```python
from build123d import *

# Parameters (mm, degrees)
SKETCH_1_W          = 120
SKETCH_1_H          = 64.5
EXTRUDE_1_DEPTH     = 44.5
SKETCH_2_W          = 24.5
SKETCH_2_H          = 24.5
CUT_EXTRUDE_1_DEPTH = 121
EXTRUDE_2_DEPTH     = 64.5
SKETCH_4_R          = 20
EXTRUDE_3_DEPTH     = 30
SKETCH_5_R          = 20
EXTRUDE_4_DEPTH     = 30
SKETCH_6_W          = 64.5
SKETCH_6_H          = 20
EXTRUDE_5_DEPTH     = 120


with BuildPart() as part:
    # 草图1 → 凸台-拉伸1 (new body)
    with BuildSketch(Plane(origin=(0, 0, 0), x_dir=(1, 0, 0), z_dir=(0, 1, 0))):
        Rectangle(SKETCH_1_W, SKETCH_1_H)
    extrude(amount=EXTRUDE_1_DEPTH)

    # 草图2 → 切除-拉伸1 (cut, through all)
    with BuildSketch(Plane(origin=(60, 0, 0), x_dir=(0, 0, -1), z_dir=(1, 0, 0))):
        with Locations((0, 12.25)):
            Rectangle(SKETCH_2_W, SKETCH_2_H)
    extrude(amount=-CUT_EXTRUDE_1_DEPTH, mode=Mode.SUBTRACT)

    # 草图3 → 凸台-拉伸2 (add)
    with BuildSketch(Plane.XY.offset(32.25)):
        with BuildLine():
            Line((-30, 44.5), (30, 44.5))
            ThreePointArc((30, 44.5), (0, 74.5), (-30, 44.5))
        make_face()
    extrude(amount=-EXTRUDE_2_DEPTH)

    # 草图4 → 凸台-拉伸3 (add)
    with BuildSketch(Plane.XY.offset(32.25)):
        with Locations((0, 44.5)):
            Circle(SKETCH_4_R)
    extrude(amount=EXTRUDE_3_DEPTH)

    # 草图5 → 凸台-拉伸4 (add)
    with BuildSketch(Plane(origin=(0, 0, -32.25), x_dir=(-1, 0, 0), z_dir=(0, 0, -1))):
        with Locations((0, 44.5)):
            Circle(SKETCH_5_R)
    extrude(amount=EXTRUDE_4_DEPTH)

    # 草图6 → 凸台-拉伸5 (add)
    with BuildSketch(Plane(origin=(60, 0, 0), x_dir=(0, 0, -1), z_dir=(1, 0, 0))):
        with Locations((0, -10)):
            Rectangle(SKETCH_6_W, SKETCH_6_H)
    extrude(amount=-EXTRUDE_5_DEPTH)


solid = part.part
```
Check sheet for the modelled part. Datum: model origin and axes. Units: mm. A direction names the side the tool comes from. Round coordinates to 2 decimals unless told otherwise and drop trailing zeros. Loops run counter-clockwise (first coordinate to the right, second up) from the corner with the lowest first, then second, coordinate; pieces in that order, holes last. Notation, with made-up numbers: M 61.5,70 L 120.5,70 A17 ccw 120.5,103 Z; hole C -32,82 d5. An arc over 180 degrees is marked long. Answer as a JSON object with one key per item and string values.
1. Access from +Z, -Z, +X, -X, +Y, -Y to the whole of each face (thin tool, end or side, straight path). Record for faces 4 (the flat face through (1, 24.5, 0)), 5 (the flat face through (-45, 44.5, 0)), 6 (the cylindrical face through (-2.6, 64.33, 47.04)).
Reply:
{"face 4": "+X, -X", "face 5": "+Z, -Z, -X, +Y", "face 6": "+Z"}
2. Gauge pin test, flat ends, axial feed: P1, Ø12, axis at x = 30.5, z = 30.5, coming from the +Y side; P2, Ø7.5, axis at x = -22.5, y = 12, coming from the -Z side; P3, Ø5, axis at x = 17, z = 39.5, coming from the +Y side (3 decimals). Record the tip position at first contact, or that the pin passes through.
Reply:
{"P1": "stops at y = 61.81", "P2": "stops at z = -32.25", "P3": "stops at y = 58.275"}
3. Section check B-B (x = 50). Record the boundary of the cut face in (y, z), plus the area to 3 significant figures.
Reply:
{"outline": "M -20,-32.25 L 44.5,-32.25 L 44.5,32.25 L -20,32.25 Z; hole M 0,-12.25 L 24.5,-12.25 L 24.5,12.25 L 0,12.25 Z", "area": "3,560 mm²"}
4. Section check C-C (x = 0). Record the boundary of the cut face in (y, z), plus the area to 4 significant figures.
Reply:
{"outline": "M -20,-32.25 L 24.5,-32.25 L 24.5,-62.25 L 64.5,-62.25 L 64.5,-32.25 L 74.5,-32.25 L 74.5,32.25 L 64.5,32.25 L 64.5,62.25 L 24.5,62.25 L 24.5,32.25 L -20,32.25 Z; hole M 0,-12.25 L 24.5,-12.25 L 24.5,12.25 L 0,12.25 Z", "area": "7,895 mm²"}
5. Section check A-A (y = 17). Record the boundary of the cut face in (x, z).
Reply:
{"outline": "M -60,-32.25 L 60,-32.25 L 60,-12.25 L -60,-12.25 Z; M -60,12.25 L 60,12.25 L 60,32.25 L -60,32.25 Z"}
6. Mould release check, pull along Y, two halves, no side actions. Record for faces 1 (the cylindrical face through (2.6, 64.33, -47.04)), 2 (the flat face through (0, 45, -62.25)), 3 (the flat face through (1, 0, 0)): pulls with the +Y half, pulls with the -Y half, needs draft (parallel to the pull), parting line crosses it, or undercut.
Reply:
{"face 1": "parting line crosses it", "face 2": "needs draft", "face 3": "undercut"}
7. Section check D-D (z = 20.5). Record the boundary of the cut face in (x, y), plus the area to 3 significant figures.
Reply:
{"outline": "M -60,-20 L 60,-20 L 60,44.5 L 30,44.5 A30 ccw -30,44.5 L -60,44.5 Z", "area": "9,150 mm²"}
8. Scan lines: line 1 (Z direction, x = -32.5, y = 17); line 2 (X direction, y = 45, z = -22); line 3 (Z direction, x = -25.5, y = 30). Record each from-to range of solid material in increasing order.
Reply:
{"line 1": "z = -32.25 to -12.25, 12.25 to 32.25", "line 2": "x = -30 to 30", "line 3": "z = -32.25 to 32.25"}
